```python
from build123d import *

# Parameters (mm, degrees)
SKETCH1_W             = 100
SKETCH1_H             = 337
SKETCH1_R             = 17
SKETCH1_R_2           = 2.5
SKETCH1_R_3           = 2
BOSS_EXTRUDE1_DEPTH   = 20
CHAMFER1_SIZE         = 45
SKETCH2_W             = 100
SKETCH2_H             = 34
CUT_EXTRUDE1_DEPTH    = 5
M4_TAPPED_HOLE1_D     = 3.3
M4_TAPPED_HOLE1_DEPTH = 16.1
M4_TAPPED_HOLE1_TIP   = 0.991420021


with BuildPart() as part:
    # Sketch1 → Boss-Extrude1 (new body)
    with BuildSketch(Plane.XY):
        with Locations((47.704546062, 452.000370419)):
            Rectangle(SKETCH1_W, SKETCH1_H)
        with Locations((65.704546062, 560.500370419)):
            Circle(SKETCH1_R, mode=Mode.SUBTRACT)
        with Locations((80.553788467, 575.349612824)):
            Circle(SKETCH1_R_2, mode=Mode.SUBTRACT)
        with Locations((80.553788467, 545.651128014)):
            Circle(SKETCH1_R_2, mode=Mode.SUBTRACT)
        with Locations((50.855303657, 545.651128014)):
            Circle(SKETCH1_R_2, mode=Mode.SUBTRACT)
        with Locations((50.855303657, 575.349612824)):
            Circle(SKETCH1_R_2, mode=Mode.SUBTRACT)
        with Locations((34.704546062, 358.500370419)):
            Circle(SKETCH1_R_3, mode=Mode.SUBTRACT)
        with Locations(Location((60.704546062, 358.500370419, 0), (0, 0, 180))):
            Circle(SKETCH1_R_3, mode=Mode.SUBTRACT)
        with Locations((60.704546062, 332.500370419)):
            Circle(SKETCH1_R_3, mode=Mode.SUBTRACT)
        with Locations(Location((34.704546062, 332.500370419, 0), (0, 0, 180))):
            Circle(SKETCH1_R_3, mode=Mode.SUBTRACT)
    extrude(amount=BOSS_EXTRUDE1_DEPTH)

    # Chamfer1
    chamfer1_edges = [part.edges().sort_by_distance(p)[0] for p in [
        (-2.295453938, 620.500370419, 10),
    ]]
    chamfer(chamfer1_edges, length=CHAMFER1_SIZE)

    # Sketch2 → Cut-Extrude1 (cut)
    with BuildSketch(Plane.XY.offset(20)):
        with Locations((47.704546062, 345.500370419)):
            Rectangle(SKETCH2_W, SKETCH2_H)
    extrude(amount=-CUT_EXTRUDE1_DEPTH, mode=Mode.SUBTRACT)

    # M4 Tapped Hole1
    with Locations(Plane(origin=(7.704546062, 283.500370419, 10), x_dir=(0, 0, -1), z_dir=(0, -1, 0))):
        with Locations((0, 0), (0, 20), (0, 60), (0, 80)):
            Hole(M4_TAPPED_HOLE1_D / 2, depth=M4_TAPPED_HOLE1_DEPTH)
            with Locations((0, 0, -(M4_TAPPED_HOLE1_DEPTH + M4_TAPPED_HOLE1_TIP / 2))):  # 118° drill point
                Cone(0, M4_TAPPED_HOLE1_D / 2, M4_TAPPED_HOLE1_TIP, mode=Mode.SUBTRACT)


solid = part.part
```
The model under review builds one solid part; all positions refer to its coordinate system, in mm. A direction names the side the tool comes from. Give positions to 0.01 mm unless a question says otherwise; leave off trailing zeros. Answer in a Markdown table with one row per item. Add a question column.
1. Wall thickness on line 1 along X through (y, z) = (290, 10); line 2 along X through (y, z) = (561, 6.75); line 3 along Y through (x, z) = (51, 14.25): over which ranges is each line inside the solid? List them lowest first. Write a range as [from, to].
2. Insertion check: P1, Ø10, axis at x = 43, y = 338.5, coming from the +Z side; P2, Ø8, axis at x = 80.55, y = 575.35, coming from the +Z side; P3, Ø2, axis at x = 87.7, z = 10, coming from the -Y side; P4, Ø12, axis at x = 22.5, z = 7.5, coming from the +Y side. Each pin has a flat end and moves straight along its axis. Give the tip position at first contact, or say it passes through.
3. Tool access review of faces 5 (the flat face through (47, 346, 15)), 6 (the flat face through (47, 283.5, 10)): name each direction out of +Z, -Z, +X, -X, +Y, -Y from which nothing blocks a thin tool from reaching the whole face with its end or side.
4. Draft analysis for pull direction X (two halves, no side actions). For faces 1 (the flat face through (97.705, 450, 10)), 2 (the flat face through (47, 493, 20)), 3 (the cylindrical face through (63.491, 577.356, 9.86)), 4 (the flat face through (-2.295, 427, 10)), state which applies: +X half, -X half, draft (parallel to the pull), parting line (faces both ways), or undercut.
Ans:
| question | item | result |
|---|---|---|
| 1 | line 1 | x = [-2.3, 6.05], [9.35, 26.05], [29.35, 66.05], [69.35, 86.05], [89.35, 97.7] |
| 1 | line 2 | x = [-2.3, 48.71], [82.7, 97.7] |
| 1 | line 3 | y = [283.5, 543.16], [548.15, 551.97], [569.03, 572.85], [577.85, 620.5] |
| 2 | P1 | stops at z = 15 |
| 2 | P2 | stops at z = 20 |
| 2 | P3 | stops at y = 299.99 |
| 2 | P4 | stops at y = 606.3 |
| 3 | face 5 | +Z, +X, -X |
| 3 | face 6 | +Z, -Z, +X, -X, -Y |
| 4 | face 1 | +X half |
| 4 | face 2 | draft |
| 4 | face 3 | undercut |
| 4 | face 4 | -X half |
